Source: CAD feature listing. Evaluate the final solid. Frame: model axes, mm. Face numbers are marked on the shaded views. Round coordinates to 2 decimals unless told otherwise and drop trailing zeros. Order: outer loops, then holes, each group sorted by start corner. A loop starts at its lowest first (then second) coordinate and runs counter-clockwise, first axis right, second up. Notation, with made-up numbers: M 87,10.5 L 98,10.5 A11 ccw 98,28.5 Z; hole C -27,42.25 d3. An arc over 180 degrees is marked long. Use one line per item in the form item = value. Start each with the question number.
Q1. Section A-A (y = 6). Return the cut outline in (x, z), plus the area to 3 significant figures.
Q2. Section B-B (x = 16.5). Return the cut outline in (y, z), plus the area to 3 significant figures.
Q3. Contact query for flat-ended pins moving along their axis: pin 1 (4.5 mm diameter, centred on x = -17, z = 47.5, fed in from +Y); pin 2 (7 mm diameter, centred on x = 16.5, z = 48.5, fed in from +Y); pin 3 (2.5 mm diameter, centred on y = 14.5, z = 48, fed in from +X). Output: stop coordinate, or through.
Q4. Section D-D (y = 2). Return the cut outline in (x, z), plus the area to 3 significant figures.
Q5. Material intervals for probe 1 along Z at (x, y) = (16.5, 7.75); probe 2 along Z at (x, y) = (16.5, 19); probe 3 along X at (y, z) = (6, 48.5), sorted ascending.
Q6. Section C-C (z = 11.5). Return the cut outline in (x, y), plus the area to 3 significant figures.
Q7. Pull-direction query (X, two-part tool) for the marked faces 1, 2 and 3; classes: pulls with the +X half, pulls with the -X half, needs draft (parallel to the pull), parting line crosses it, or undercut.
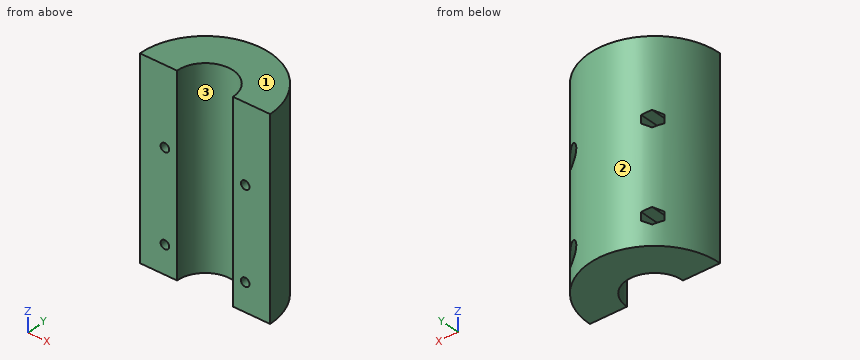
from build123d import *

# Parameters (mm, degrees)
F1_DEPTH       = 80
F4_D           = 3.5
F4_START       = 9.5653412
F4_CBORE_D     = 8
F4_CBORE_DEPTH = 7
F5_D           = 3.5
F6_DEPTH       = 25
F7_DEPTH       = 14


with BuildPart() as f1:
    # F0 (on Top) → F1 (new body)
    with BuildSketch(Plane.XY):
        with BuildLine():
            Line((11.4989534177, -0.1551460505), (26.7495500841, -0.1551460505))
            ThreePointArc((26.7495500841, -0.1551460505), (0, 26.75), (-26.7495500841, -0.1551460505))
            Line((-26.7495500841, -0.1551460505), (-11.4989534177, -0.1551460505))
            ThreePointArc((-11.4989534177, -0.1551460505), (0, 11.5), (11.4989534177, -0.1551460505))
        make_face()
    extrude(amount=F1_DEPTH)

    # F4 (through all)
    # its depths count from where the whole tool has entered the part; down to there all is cleared
    with Locations(Plane(origin=(0, 26.75, 0), x_dir=(1, 0, 0), z_dir=(0, 1, 0)).offset(-F4_START)):
        with Locations((16.5, -48.5), (16.5, -11.5)):
            CounterBoreHole(F4_D / 2, F4_CBORE_D / 2, F4_CBORE_DEPTH)

    # F5 (through all)
    with Locations(Plane(origin=(0, 26.75, 0), x_dir=(1, 0, 0), z_dir=(0, 1, 0))):
        with Locations((-16.5, -48.5), (-16.5, -11.5)):
            Hole(F5_D / 2)

    # F3 (on offset) → F6 (cut)
    with BuildSketch(Plane.XZ.offset(-26.75)):
        Polygon((-16.5, 45.1513684387), (-13.6, 46.8256842194), (-13.6, 50.1743157806), (-16.5, 51.8486315613), (-19.4, 50.1743157806), (-19.4, 46.8256842194), align=None)
    extrude(amount=-F6_DEPTH, mode=Mode.SUBTRACT)

    # F3 (on offset) → F7 (cut)
    with BuildSketch(Plane.XZ.offset(-26.75)):
        Polygon((-16.5, 45.1513684387), (-13.6, 46.8256842194), (-13.6, 50.1743157806), (-16.5, 51.8486315613), (-19.4, 50.1743157806), (-19.4, 46.8256842194), align=None)
        Polygon((-16.5, 8.1513684387), (-13.6, 9.8256842194), (-13.6, 13.1743157806), (-16.5, 14.8486315613), (-19.4, 13.1743157806), (-19.4, 9.8256842194), align=None)
    extrude(amount=F7_DEPTH, mode=Mode.SUBTRACT)


solid = f1.part
Results list:
q1.outline = M -26.07,0 L -9.81,0 L -9.81,80 L -26.07,80 Z; M 9.81,0 L 26.07,0 L 26.07,80 L 9.81,80 Z; hole C -16.5,11.5 d3.5; hole C -16.5,48.5 d3.5; hole C 16.5,11.5 d3.5; hole C 16.5,48.5 d3.5
q1.area = 2,560 mm2
q2.outline = M -0.16,0 L 21.05,0 L 21.05,7.5 L 10.18,7.5 L 10.18,9.75 L -0.16,9.75 Z; M -0.16,13.25 L 10.18,13.25 L 10.18,15.5 L 21.05,15.5 L 21.05,44.5 L 10.18,44.5 L 10.18,46.75 L -0.16,46.75 Z; M -0.16,50.25 L 10.18,50.25 L 10.18,52.5 L 21.05,52.5 L 21.05,80 L -0.16,80 Z
q2.area = 1,450 mm2
q3.pin_1 = 20.89
q3.pin_2 = 10.18
q3.pin_3 = 23.24
q4.outline = M -26.68,0 L -11.32,0 L -11.32,80 L -26.68,80 Z; M 11.32,0 L 26.68,0 L 26.68,80 L 11.32,80 Z; hole C -16.5,11.5 d3.5; hole C -16.5,48.5 d3.5; hole C 16.5,11.5 d3.5; hole C 16.5,48.5 d3.5
q4.area = 2,420 mm2
q5.probe_1 = 0 to 9.75, 13.25 to 46.75, 50.25 to 80
q5.probe_2 = 0 to 7.5, 15.5 to 44.5, 52.5 to 80
q5.probe_3 = -26.07 to -18.25, -14.75 to -9.81, 9.81 to 14.75, 18.25 to 26.07
q6.outline = M -26.75,-0.16 L -18.25,-0.16 L -18.25,12.75 L -19.4,12.75 L -19.4,18.42 A26.75 ccw Z; M -14.75,-0.16 L -11.5,-0.16 A11.5 cw long 11.5,-0.16 L 14.75,-0.16 L 14.75,10.18 L 12.5,10.18 L 12.5,23.65 A26.75 ccw -13.6,23.03 L -13.6,12.75 L -14.75,12.75 Z; M 18.25,-0.16 L 26.75,-0.16 A26.75 ccw 20.5,17.18 L 20.5,10.18 L 18.25,10.18 Z
q6.area = 707 mm2
q7.face_1 = needs draft
q7.face_2 = parting line crosses it
q7.face_3 = undercut
